from build123d import *

# Parameters (mm, degrees)
BOSS_EXTRUDE1_DEPTH     = 7.7
SKETCH2_W               = 7
SKETCH2_H               = 3.1
CUT_EXTRUDE1_DEPTH      = 79.027559234
FILLET1_R               = 10
BOSS_EXTRUDE2_DEPTH     = 2
BOSS_EXTRUDE3_DEPTH     = 33.45
BOSS_EXTRUDE4_REACH     = 112.929
CUT_EXTRUDE2_DEPTH      = 111.928772192
CUT_EXTRUDE2_DEPTH_BACK = 111.928772192
CUT_EXTRUDE3_DEPTH      = 10
FILLET3_R               = 1
FILLET5_R               = 3
SKETCH8_W               = 17
SKETCH8_H               = 5
CUT_EXTRUDE4_DEPTH      = 2
FILLET6_R               = 5
FILLET7_R               = 2


with BuildPart() as part:
    # Sketch1 → Boss-Extrude1 (new body)
    with BuildSketch(Plane(origin=(0, 0, 0), x_dir=(1, 0, 0), z_dir=(0, 1, 0))):
        Polygon((0, 0), (-16.35, 0), (-16.35, -9.85), (-2.6, -9.85), (-2.6, -33), (-20.1, -33), (-20.1, -75), (0, -75), align=None)
    extrude(amount=BOSS_EXTRUDE1_DEPTH)

    # Sketch2 → Cut-Extrude1 (cut, through all)
    with BuildSketch(Plane.XY.offset(75)):
        with Locations((-16.6, 3.55)):
            Rectangle(SKETCH2_W, SKETCH2_H)
    extrude(amount=-CUT_EXTRUDE1_DEPTH, mode=Mode.SUBTRACT)

    # Fillet1
    fillet1_edges = [part.edges().sort_by_distance(p)[0] for p in [
        (-2.6, 3.85, 33),
    ]]
    fillet(fillet1_edges, radius=FILLET1_R)

    # Sketch3 → Boss-Extrude2 (add)
    with BuildSketch(Plane(origin=(0, 7.7, 0), x_dir=(1, 0, 0), z_dir=(0, 1, 0))):
        Polygon((0, 4.5), (-33.45, 4.5), (-33.45, -75), (-10, -105), (0, -105), align=None)
    extrude(amount=BOSS_EXTRUDE2_DEPTH)

    # Sketch4 → Boss-Extrude3 (add)
    with BuildSketch(Plane(origin=(0, 0, 0), x_dir=(0, 0, -1), z_dir=(1, 0, 0))):
        Polygon((-105, 9.7), (-105, 12.7), (-90, 12.7), (-50.25, 9.7), align=None)
    extrude(amount=-BOSS_EXTRUDE3_DEPTH)

    # Boss-Extrude4: up to this face of the body (flat: up to its plane)
    boss_extrude4_end = Plane(part.part.faces().sort_by_distance((0, 5.848980441, 46.191947566))[0])
    # Sketch5 → Boss-Extrude4 (add, up to the picked face)
    with BuildSketch(Plane.ZY.offset(33.45), mode=Mode.PRIVATE) as boss_extrude4_sk1:
        Polygon((75, 7.7), (75, -5), (82, -5), (105, 7.7), align=None)
    boss_extrude4_tool1 = split(extrude(boss_extrude4_sk1.sketch, amount=-BOSS_EXTRUDE4_REACH, mode=Mode.PRIVATE), bisect_by=boss_extrude4_end, keep=Keep.BOTH, mode=Mode.PRIVATE)
    add(boss_extrude4_tool1.solids().sort_by(Axis((-33.45, 2.665766, 85.441441), (1, 0, 0)))[0])

    # Sketch6 → Cut-Extrude2 (cut, two sides: drawn at the far end of the back side and taken through both)
    with BuildSketch(Plane(origin=(0, 7.7, 0), x_dir=(1, 0, 0), z_dir=(0, 1, 0)).offset(-CUT_EXTRUDE2_DEPTH_BACK)):
        Polygon((-33.45, -75), (-10, -105), (-33.45, -105), align=None)
    extrude(amount=CUT_EXTRUDE2_DEPTH + CUT_EXTRUDE2_DEPTH_BACK, mode=Mode.SUBTRACT)

    # Sketch7 → Cut-Extrude3 (cut)
    with BuildSketch(Plane(origin=(0, 0, 0), x_dir=(0, 0, -1), z_dir=(1, 0, 0))):
        Polygon((-75, 0), (-85, 0), (-80, -5), (-75, -5), align=None)
    extrude(amount=-CUT_EXTRUDE3_DEPTH, mode=Mode.SUBTRACT)

    # Fillet3
    # the kernel refuses this fillet: 1 mm, written as the material it takes off along each edge
    with BuildSketch(Plane(origin=(5.810983209, -5, 80), x_dir=(0, 0, 1), z_dir=(-1, 0, 0))) as fillet3_piece_1:
        with BuildLine():
            CenterArc((2.350701034, 0.936487472), FILLET3_R, 135, 114.469800521)
            Line((1.643594253, 1.643594253), (1.629452117, 1.657736389))
            Line((1.629452117, 1.657736389), (-0.014142136, 0.014142136))
            Line((-0.014142136, 0.014142136), (0, -0.02))
            ThreePointArc((0, -0.02), (1, -0.02), (1.992985979, -0.018729749))
            Line((1.992985979, -0.018729749), (2, 0))
        make_face()
    extrude(amount=15.810983209, mode=Mode.SUBTRACT)
    with BuildSketch(Plane(origin=(-10, -5, 82.5), x_dir=(-1, 0, 0), z_dir=(0, 0, -1))) as fillet3_piece_2_section:
        with BuildLine():
            CenterArc((FILLET3_R, FILLET3_R), FILLET3_R, 180, 90)
            Line((0, FILLET3_R), (-FILLET3_R * 0.02, FILLET3_R))
            Line((-FILLET3_R * 0.02, FILLET3_R), (-FILLET3_R * 0.02, -FILLET3_R * 0.02))
            Line((-FILLET3_R * 0.02, -FILLET3_R * 0.02), (FILLET3_R, -FILLET3_R * 0.02))
            Line((FILLET3_R, -FILLET3_R * 0.02), (FILLET3_R, 0))
        make_face()
    fillet3_piece_2 = extrude(amount=10, mode=Mode.PRIVATE)
    fillet3_piece_2 = split(fillet3_piece_2, bisect_by=Plane(origin=(-10.222841489, -6.700692184, 78.299307816), z_dir=(0, 0.7071067811865466, -0.7071067811865485)), keep=Keep.TOP, mode=Mode.PRIVATE)
    add(fillet3_piece_2, mode=Mode.SUBTRACT)
    with BuildSketch(Plane(origin=(5.810983209, -5, 80), x_dir=(0, 0, 1), z_dir=(-1, 0, 0))) as fillet3_piece_3a_section:
        with BuildLine():
            CenterArc((2.350701034, 0.936487472), FILLET3_R, 135, 114.469800521)
            Line((1.643594253, 1.643594253), (1.629452117, 1.657736389))
            Line((1.629452117, 1.657736389), (-0.014142136, 0.014142136))
            Line((-0.014142136, 0.014142136), (0, -0.02))
            ThreePointArc((0, -0.02), (1, -0.02), (1.992985979, -0.018729749))
            Line((1.992985979, -0.018729749), (2, 0))
        make_face()
    fillet3_piece_3a = extrude(amount=21.621966417, mode=Mode.PRIVATE)
    fillet3_piece_3a = split(fillet3_piece_3a, bisect_by=Plane(origin=(-10, -4.567151235, 80.996776665), z_dir=(-1, 0, 0)), keep=Keep.TOP, mode=Mode.PRIVATE)
    with BuildSketch(Plane(origin=(-10, -5, 82.5), x_dir=(-1, 0, 0), z_dir=(0, 0, -1))) as fillet3_piece_3b_section:
        with BuildLine():
            CenterArc((FILLET3_R, FILLET3_R), FILLET3_R, 180, 90)
            Line((0, FILLET3_R), (-FILLET3_R * 0.02, FILLET3_R))
            Line((-FILLET3_R * 0.02, FILLET3_R), (-FILLET3_R * 0.02, -FILLET3_R * 0.02))
            Line((-FILLET3_R * 0.02, -FILLET3_R * 0.02), (FILLET3_R, -FILLET3_R * 0.02))
            Line((FILLET3_R, -FILLET3_R * 0.02), (FILLET3_R, 0))
        make_face()
    fillet3_piece_3b = extrude(amount=10, mode=Mode.PRIVATE)
    fillet3_piece_3b = split(fillet3_piece_3b, bisect_by=Plane(origin=(-10.238471404, -4.220535034, 80.779464966), z_dir=(0, -0.7071067811865466, 0.7071067811865485)), keep=Keep.TOP, mode=Mode.PRIVATE)
    fillet3_piece_3 = fillet3_piece_3a & fillet3_piece_3b
    add(fillet3_piece_3, mode=Mode.SUBTRACT)

    # Mirror1: part across plane


with BuildPart() as part_1:
    add(part.part)
    add(part.part.mirror(Plane(origin=(0, 7.7, 75), x_dir=(0, 0, 1), z_dir=(-1, 0, 0))))

    # Fillet5
    # the kernel refuses this fillet: 3 mm, written as the material it takes off along each edge
    with BuildSketch(Plane(origin=(-38.068859068, -5, 69.091011854), x_dir=(0, 1, 0), z_dir=(0.6158478756904763, 0, 0.7878650861711843)), Plane(origin=(38.068859068, -5, 69.091011854), x_dir=(-0.7878650861711843, 0, -0.6158478756904764), z_dir=(-0.6158478756904763, 0, 0.7878650861711843))) as fillet5_piece_1:
        with BuildLine():
            CenterArc((FILLET5_R, -FILLET5_R), FILLET5_R, 90, 90)
            Line((0, -FILLET5_R), (0, 0))
            Line((0, 0), (FILLET5_R, 0))
        make_face()
    extrude(amount=23.884769896, mode=Mode.SUBTRACT)

    # Sketch8 → Cut-Extrude4 (cut)
    with BuildSketch(Plane(origin=(0, 9.7, 0), x_dir=(1, 0, 0), z_dir=(0, 1, 0))):
        with Locations((24.95, 2)):
            Rectangle(SKETCH8_W, SKETCH8_H)
    extrude(amount=-CUT_EXTRUDE4_DEPTH, mode=Mode.SUBTRACT)

    # Fillet6
    fillet6_edges = [part_1.edges().sort_by_distance(p)[0] for p in [
        (-33.45, 8.7, -4.5),
    ]]
    fillet(fillet6_edges, radius=FILLET6_R)

    # Fillet7
    fillet7_edges = [part_1.edges().sort_by_distance(p)[0] for p in [
        (16.45, 8.7, -4.5),
        (33.45, 8.7, 0.5),
    ]]
    fillet(fillet7_edges, radius=FILLET7_R)


solid = part_1.part
Could you check a few things on this model? Use its own coordinates, in mm. A direction names the side the tool comes from. Coordinates: 2 decimals unless noted, no trailing zeros. Order: outer loops, then holes, each group sorted by start corner. A loop starts at its lowest first (then second) coordinate and runs counter-clockwise, first axis right, second up.
Q1. Suppose I cut it at C-C on z = 35.5. Please give me the cut outline in (x, y).
Q2. Suppose I cut it at B-B on x = 6.5. Please give me the cut outline in (y, z), and give its area (3 significant figures).
Q3. Will these pins go through, and if not, where does the flat tip stop? pin 1 (0.8 mm diameter, centred on y = 6, z = 6, fed in from +X); pin 2 (2 mm diameter, centred on y = 7, z = 51, fed in from +X); pin 3 (0.9 mm diameter, centred on y = 3.5, z = 45.5, fed in from +X); pin 4 (4 mm diameter, centred on x = -11, y = 4.5, fed in from +Z).
Q4. Thinking about a two-plate mould opening in Y: for faces 1 (the flat face through (-17, 5.1, 54)), 2 (the cylindrical face through (-31.95, 8.71, -3.07)), 3 (the flat face through (-18, -5, 78)), which applies, released by +Y, released by -Y, zero draft, split by the parting line, or undercut?
Q5. Suppose I cut it at A-A on z = 8. Please give me the cut outline in (x, y).
Q6. Which directions (+Z, -Z, +X, -X, +Y, -Y) give clear straight access to the entire face, cutting with the end or side of a thin tool? Please do faces 4 (the flat face through (16.45, 9, -1)), 5 (the flat face through (0, 4, 0)), 6 (the flat face through (15, 2, 5)).
Q7. Please list where these lines run through material, in increasing order: L1, parallel to Y at x = 22, z = 18; L2, parallel to Y at x = -9.5, z = 9; L3, parallel to Y at x = 9.5, z = 81.5.
Q8. Suppose I cut it at D-D on x = 19. Please give me the cut outline in (y, z).
Answer:
1. outline: (-33.45, 7.7) - (-20.1, 7.7) - (-20.1, 5.1) - (-13.1, 5.1) - (-13.1, 2) - (-20.1, 2) - (-20.1, 0) - (20.1, 0) - (20.1, 2) - (13.1, 2) - (13.1, 5.1) - (20.1, 5.1) - (20.1, 7.7) - (33.45, 7.7) - (33.45, 9.7) - (-33.45, 9.7) - close
2. outline: (-5, 82) arc R1 ccw to (-3.36, 81.64) - (0, 85) - (0, 30.92) - (7.7, 30.92) - (7.7, 9.85) - (0, 9.85) - (0, 0) - (7.7, 0) - (7.7, -4.5) - (9.7, -4.5) - (9.7, 50.25) - (12.7, 90) - (12.7, 105) - (7.7, 105) - close
2. area: 935 mm2
3. pin 1: stops at x = 16.35
3. pin 2: stops at x = 33.45
3. pin 3: stops at x = 13.1
3. pin 4: stops at z = 102.83
4. face 1: undercut
4. face 2: zero draft
4. face 3: released by -Y
5. outline: (-33.45, 7.7) - (-16.35, 7.7) - (-16.35, 5.1) - (-13.1, 5.1) - (-13.1, 2) - (-16.35, 2) - (-16.35, 0) - (16.35, 0) - (16.35, 2) - (13.1, 2) - (13.1, 5.1) - (16.35, 5.1) - (16.35, 7.7) - (33.45, 7.7) - (33.45, 9.7) - (-33.45, 9.7) - close
6. face 4: -Z, +X, +Y, -Y
6. face 5: -Z, +X, -X, -Y
6. face 6: -Z, +X
7. L1: y = 7.7 to 9.7
7. L2: y = 0 to 9.7
7. L3: y = -4.59 to -3.54, 0 to 12.06
8. outline: (-5, 75) - (0, 75) - (0, 33) - (2, 33) - (2, 75) - (5.1, 75) - (5.1, 33) - (7.7, 33) - (7.7, 0.5) - (9.7, 0.5) - (9.7, 50.25) - (12.7, 90) - (12.7, 93.49) - (1.34, 93.49) - (-5, 82) - close
